The listing builds one solid part. Answer for the finished solid, in the listing's coordinates (mm). Face numbers are marked on the shaded views. A direction names the side the tool comes from. Give positions to 0.01 mm unless a question says otherwise; leave off trailing zeros. Write each loop counter-clockwise with the first axis right and the second up, starting at its lowest first coordinate (ties: lowest second). Pieces come first, ordered by that corner, then holes. Notation, with made-up numbers: M 17,62.25 L 72,62.25 A14 cw 72,83.25 Z; hole C 1.25,-38 d10. An arc over 180 degrees is marked long. Answer as a JSON object with one key per item and string values.
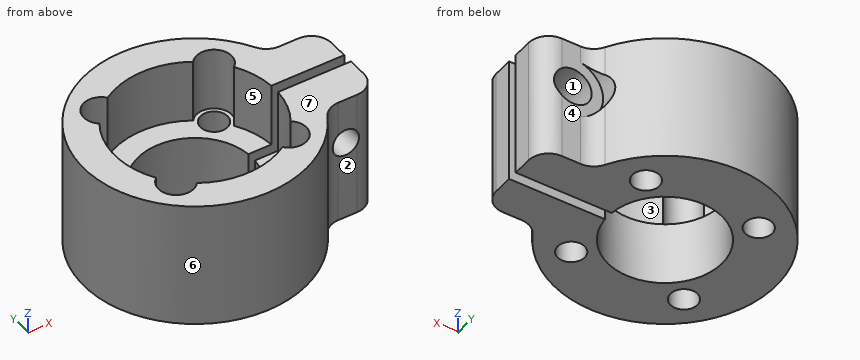
```python
from build123d import *

# Parameters (mm, degrees)
BOSS_EXTRUDE1_DEPTH       = 6.35
F_6_32_TAPPED_HOLE3_D     = 2.7051
SKETCH14_R                = 1.85
CUT_EXTRUDE6_DEPTH        = 21.223068511
F_6_32_TAPPED_HOLE5_D     = 2.7051
F_6_32_TAPPED_HOLE5_DEPTH = 50.8
F_6_32_TAPPED_HOLE5_TIP   = 0.81269403
SKETCH24_R                = 3
CUT_EXTRUDE26_DEPTH       = 36.126165479
FILLET1_R                 = 2
SKETCH28_R                = 1.75
CUT_EXTRUDE27_DEPTH       = 6.35


with BuildPart() as part:
    # Sketch1 → Boss-Extrude1 (new, symmetric)
    with BuildSketch(Plane.XY):
        with BuildLine():
            Line((0, 0), (0, 0.5))
            Line((0, 0.5), (15.3, 0.5))
            Line((15.3, 0.5), (15.3, 4.45))
            Line((15.3, 4.45), (11.402083143, 4.45))
            ThreePointArc((11.402083143, 4.45), (10.394478471, 4.722362068), (9.661307091, 5.465267176))
            ThreePointArc((9.661307091, 5.465267176), (-11.1, 0), (9.661307091, -5.465267176))
            ThreePointArc((9.661307091, -5.465267176), (10.394478471, -4.722362068), (11.402083143, -4.45))
            Line((11.402083143, -4.45), (15.3, -4.45))
            Line((15.3, -4.45), (15.3, -0.5))
            Line((15.3, -0.5), (0, -0.5))
            Line((0, -0.5), (0, 0))
        make_face()
    extrude(amount=BOSS_EXTRUDE1_DEPTH, both=True)

    # Sketch27 → Cut-Revolve1 (revolve, cut)
    with BuildSketch(Plane(origin=(0, 0, 0), x_dir=(1, 0, 0), z_dir=(0, 1, 0))):
        Polygon((0, 6.35), (5.7, 6.35), (5.7, 0), (8, 0), (8, -6.35), (0, -6.35), align=None)
    revolve(axis=Axis((0, 0, -6.35), (0, 0, 1)), mode=Mode.SUBTRACT)

    # #6-32 Tapped Hole3 (through all)
    with Locations(Plane(origin=(-5.656516225, 5.657192254, -6.35), x_dir=(-1, 0, 0), z_dir=(0, 0, -1))):
        with Locations((0, 0), (-11.313708479, -0.000676029), (-11.31303245, -11.314384508), (0.000676029, -11.313708479)):
            Hole(F_6_32_TAPPED_HOLE3_D / 2)

    # Sketch14 → Cut-Extrude6 (cut, through all)
    with BuildSketch(Plane.XZ.offset(-0.5)):
        with Locations(Location((12.15, 1.7, 0), (0, 0, 270))):
            Circle(SKETCH14_R)
    extrude(amount=-CUT_EXTRUDE6_DEPTH, mode=Mode.SUBTRACT)

    # #6-32 Tapped Hole5
    with Locations(Plane(origin=(0, -0.5, 0), x_dir=(-1, 0, 0), z_dir=(0, 1, 0))):
        with Locations((-12.15, 1.7)):
            Hole(F_6_32_TAPPED_HOLE5_D / 2, depth=F_6_32_TAPPED_HOLE5_DEPTH)
            with Locations((0, 0, -(F_6_32_TAPPED_HOLE5_DEPTH + F_6_32_TAPPED_HOLE5_TIP / 2))):  # 118° drill point
                Cone(0, F_6_32_TAPPED_HOLE5_D / 2, F_6_32_TAPPED_HOLE5_TIP, mode=Mode.SUBTRACT)

    # Sketch24 → Cut-Extrude26 (cut, through all)
    with BuildSketch(Plane(origin=(19.75, 4.45, 0), x_dir=(0, 0, -1), z_dir=(0, 1, 0))):
        with Locations((-1.7, 7.6)):
            Circle(SKETCH24_R)
    extrude(amount=CUT_EXTRUDE26_DEPTH, mode=Mode.SUBTRACT)

    # Fillet1
    # the kernel refuses this fillet: 2 mm, written as the material it takes off along each edge
    with BuildSketch(Plane(origin=(15.3, -4.45, -11.35), x_dir=(0, 1, 0), z_dir=(0, 0, 1))) as fillet1_piece_1:
        with BuildLine():
            CenterArc((FILLET1_R, FILLET1_R), FILLET1_R, 180, 90)
            Line((0, FILLET1_R), (0, 0))
            Line((0, 0), (FILLET1_R, 0))
        make_face()
    extrude(amount=22.7, mode=Mode.SUBTRACT)
    with BuildSketch(Plane(origin=(15.3, 4.45, -11.35), x_dir=(0, -1, 0), z_dir=(0, 0, 1))) as fillet1_piece_2:
        with BuildLine():
            CenterArc((FILLET1_R, -FILLET1_R), FILLET1_R, 90, 90)
            Line((0, -FILLET1_R), (0, 0))
            Line((0, 0), (FILLET1_R, 0))
        make_face()
    extrude(amount=22.7, mode=Mode.SUBTRACT)

    # Sketch28 → Cut-Extrude27 (cut)
    with BuildSketch(Plane.XY.offset(6.35)):
        with Locations((5.656516225, -5.657192254)):
            Circle(SKETCH28_R)
        with Locations((-5.656516225, 5.657192254)):
            Circle(SKETCH28_R)
        with Locations((5.657192254, 5.656516225)):
            Circle(SKETCH28_R)
        with Locations((-5.657192254, -5.656516225)):
            Circle(SKETCH28_R)
    extrude(amount=-CUT_EXTRUDE27_DEPTH, mode=Mode.SUBTRACT)


solid = part.part
```
1. A cutting plane is placed at B-B, the plane x = 0. Give the vertices of the cut face in (y, z).
Verdict:
{"outline": "M -11.1,-6.35 L -5.7,-6.35 L -5.7,0 L -8,0 L -8,6.35 L -11.1,6.35 Z; M 5.7,-6.35 L 11.1,-6.35 L 11.1,6.35 L 8,6.35 L 8,0 L 5.7,0 Z"}
2. For the marked faces 1, 2, 3 and 4, determine the directions among +Z, -Z, +X, -X, +Y, -Y from which every point of the face is accessible in a straight line to the end or side of a thin tool.
Verdict:
{"face 1": "+Y", "face 2": "+Z, -Z, +X, -Y", "face 3": "+Z", "face 4": "+X, +Y"}
3. A cutting plane is placed at D-D, the plane z = 1.7. Give the vertices of the cut face in (x, y), plus the area to 3 significant figures.
Verdict:
{"outline": "M -6.75,-4.29 A8 cw -6.75,4.29 A1.75 cw long -4.29,6.75 A8 cw 4.29,6.75 A1.75 cw long 6.75,4.29 A8 cw 7.98,0.5 L 10.3,0.5 L 10.3,4.45 L 9.15,4.45 L 9.15,6.28 A11.1 ccw long 9.66,-5.47 A2 cw 10.8,-4.54 L 10.8,-0.5 L 7.98,-0.5 A8 cw 6.75,-4.29 A1.75 cw long 4.29,-6.75 A8 cw -4.29,-6.75 A1.75 cw long Z; M 13.5,-4.44 A2 ccw 15.3,-2.45 L 15.3,-0.5 L 13.5,-0.5 Z; M 14,0.5 L 15.3,0.5 L 15.3,2.45 A2 ccw 14,4.32 Z", "area": "171 mm2"}
4. The mould has two halves that part along X. Classify the marked faces 5, 6 and 7: released by +X, released by -X, zero draft, split by the parting line, or undercut.
Verdict:
{"face 5": "undercut", "face 6": "split by the parting line", "face 7": "zero draft"}
5. Consider line 1 along Y through (x, z) = (7.25, 5.25); line 2 along Y through (x, z) = (0.25, 5); line 3 along Y through (x, z) = (0, -2.75). Determine where each line is inside the solid, lowest interval first.
Verdict:
{"line 1": "y = -8.41 to -6.38, -4.93 to -3.38, 3.38 to 4.93, 6.38 to 8.41", "line 2": "y = -11.1 to -8, 8 to 11.1", "line 3": "y = -11.1 to -5.7, 5.7 to 11.1"}
6. Flat-ended cylindrical pins translate along their axes: pin 1 (4.5 mm diameter, centred on x = 12.15, z = 1.7, fed in from -Y); pin 2 (2 mm diameter, centred on x = 12.5, z = 3.5, fed in from -Y); pin 3 (7.5 mm diameter, centred on x = 10.5, z = 0, fed in from +Y). Find the tip coordinate at first contact, or state that the pin passes through.
Verdict:
{"pin 1": "stops at y = -5.13", "pin 2": "stops at y = -4.45", "pin 3": "stops at y = 8.81"}
7. A cutting plane is placed at A-A, the plane x = 12.15. Give the vertices of the cut face in (y, z).
Verdict:
{"outline": "M -4.45,-6.35 L -0.5,-6.35 L -0.5,0.35 L -4.45,0.35 Z; M -4.45,3.05 L -0.5,3.05 L -0.5,6.35 L -4.45,6.35 Z; M 0.5,-6.35 L 4.45,-6.35 L 4.45,-0.15 L 0.5,-0.15 Z; M 0.5,3.55 L 4.45,3.55 L 4.45,6.35 L 0.5,6.35 Z"}
8. A cutting plane is placed at C-C, the plane y = 2. Give the vertices of the cut face in (x, z).
Verdict:
{"outline": "M -10.92,-6.35 L -5.34,-6.35 L -5.34,0 L -7.75,0 L -7.75,6.35 L -10.92,6.35 Z; M 5.34,-6.35 L 15.3,-6.35 L 15.3,6.35 L 7.75,6.35 L 7.75,0 L 5.34,0 Z; hole C 12.15,1.7 d3.7"}
